The listing builds one solid part. Answer for the finished solid, in the listing's coordinates (mm). A direction names the side the tool comes from. Coordinates: 2 decimals unless noted, no trailing zeros. Loops run counter-clockwise (first coordinate to the right, second up) from the corner with the lowest first, then second, coordinate; pieces in that order, holes last. Notation, with made-up numbers: (-14, 72) - (18, 72) arc R24 ccw to (18, 99) - close; hole circle Ø2 at (37, 55). An arc over 180 degrees is marked (long way). Put each result on its own line as item: value.
```python
from build123d import *

# Parameters (mm, degrees)
SKETCH1_W                = 100
SKETCH1_H                = 101.866666666
BOSS_EXTRUDE1_DEPTH      = 100
BOSS_EXTRUDE2_DEPTH      = 300
BOSS_EXTRUDE2_DEPTH_BACK = 400
SKETCH2_W                = 10
SKETCH2_H                = 75
EXTRUDE_THIN1_START      = -20
EXTRUDE_THIN1_DEPTH      = 40


# Read off the part's stored shape, not the designer's step: Extrude-Thin1
with BuildPart() as part:
    # Sketch1 → Boss-Extrude1 (new body)
    with BuildSketch(Plane.XY):
        Rectangle(SKETCH1_W, SKETCH1_H)
    extrude(amount=BOSS_EXTRUDE1_DEPTH)

    # Sketch2 → Boss-Extrude2 (add, two sides: drawn at the far end of the back side and taken through both)
    with BuildSketch(Plane(origin=(50, 0, 0), x_dir=(0, 0, -1), z_dir=(1, 0, 0)).offset(-BOSS_EXTRUDE2_DEPTH_BACK)):
        with Locations((-50, 0.933333333)):
            Rectangle(SKETCH2_W, SKETCH2_H)
    extrude(amount=BOSS_EXTRUDE2_DEPTH + BOSS_EXTRUDE2_DEPTH_BACK)

    # Extrude-Thin1 outline → Extrude-Thin1 (add)
    with BuildSketch(Plane.XY.offset(50).offset(EXTRUDE_THIN1_START)):
        with BuildLine():
            Line((5, 50.933333333), (5, 72.767361549))
            ThreePointArc((5, 72.767361549), (55.2653102, 133.511715936), (58.591267344, 212.286178857))
            Line((58.591267344, 212.286178857), (48.987221146, 209.500089011))
            ThreePointArc((48.987221146, 209.500089011), (45.987027323, 137.245454908), (0, 81.433927153))
            ThreePointArc((0, 81.433927153), (-45.987027323, 137.245454908), (-48.987221146, 209.500089011))
            Line((-48.987221146, 209.500089011), (-58.591267344, 212.286178857))
            ThreePointArc((-58.591267344, 212.286178857), (-55.2653102, 133.511715936), (-5, 72.767361549))
            Line((-5, 72.767361549), (-5, 50.933333333))
            Line((-5, 50.933333333), (5, 50.933333333))
        make_face()
    extrude(amount=EXTRUDE_THIN1_DEPTH)


solid = part.part
```
1) Straight lines are drawn through the part: L1, parallel to Y at x = -24, z = 84; L2, parallel to Z at x = 172, y = -5; L3, parallel to X at y = 70, z = 33. For each, find the intervals that lie inside material, in ascending order. Write a range as [from, to].
Found:
L1: y = [-50.93, 50.93]
L2: z = [45, 55]
L3: x = [-5, 5]
2) Each of these flat-tipped pins is pushed along its axis until it touches: pin 1 (5 mm diameter, centred on x = -165.5, z = 47.5, fed in from -Y); pin 2 (24 mm diameter, centred on y = 65, z = 40.5, fed in from +X); pin 3 (11 mm diameter, centred on y = 58.5, z = 47.5, fed in from -X). Where does it stop, or does it pass through?
Found:
pin 1: stops at y = -36.57
pin 2: stops at x = 11.38
pin 3: stops at x = -5
3) For a pull along X with two mould halves and no side action, classify faces 4 (the face through (-38, 120, 30)), 5 (the face through (5, 62, 50)), 6 (the face through (-45.615, 136.285, 49.72)), 7 (the face through (46.35, 138.21, 49.72)) as pulls with the +X half, pulls with the -X half, needs draft (parallel to the pull), parting line crosses it, or undercut.
Found:
face 4: needs draft
face 5: pulls with the +X half
face 6: undercut
face 7: undercut
4) The part is cut by section B-B (x = 17). Give the vertices of the cut face in (y, z).
Found:
outline: (-50.93, 0) - (50.93, 0) - (50.93, 100) - (-50.93, 100) - close; (81.23, 30) - (94.41, 30) - (94.41, 70) - (81.23, 70) - close
5) The part is cut by section D-D (z = 37.5). Give the vertices of the cut face in (x, y).
Found:
outline: (-58.59, 212.29) arc R123.63 ccw to (-5, 72.77) - (-5, 50.93) - (-50, 50.93) - (-50, -50.93) - (50, -50.93) - (50, 50.93) - (5, 50.93) - (5, 72.77) arc R123.63 ccw to (58.59, 212.29) - (48.99, 209.5) arc R113.63 cw to (0, 81.43) arc R113.63 cw to (-48.99, 209.5) - close
6) The part is cut by section C-C (y = 149). Give the vertices of the cut face in (x, z), and give its area (3 significant figures).
Found:
outline: (-60.08, 30) - (-49.77, 30) - (-49.77, 70) - (-60.08, 70) - close; (49.77, 30) - (60.08, 30) - (60.08, 70) - (49.77, 70) - close
area: 825 mm^2
7) The part is cut by section A-A (y = 26). Give the vertices of the cut face in (x, z), and give its area (3 significant figures).
Found:
outline: (-350, 45) - (-50, 45) - (-50, 0) - (50, 0) - (50, 45) - (350, 45) - (350, 55) - (50, 55) - (50, 100) - (-50, 100) - (-50, 55) - (-350, 55) - close
area: 16,000 mm^2
8) For faces 1 (the face through (-1, 1, 0)), 2 (the face through (-38, 120, 70)), 3 (the face through (-5, 62, 50)), determine the directions among +Z, -Z, +X, -X, +Y, -Y from which every point of the face is accessible in a straight line to the end or side of a thin tool.
Found:
face 1: -Z, +X, -X, +Y, -Y
face 2: +Z, +X, -X, +Y
face 3: +Z, -Z, -X
